Source: CAD feature listing. Evaluate the final solid. Frame: model axes, mm. A direction names the side the tool comes from. Coordinates: 2 decimals unless noted, no trailing zeros. Write each loop counter-clockwise with the first axis right and the second up, starting at its lowest first coordinate (ties: lowest second). Pieces come first, ordered by that corner, then holes. Notation, with made-up numbers: M 6,74 L 65,74 A19 cw 65,110 Z; hole C -15,11 d2. An arc over 180 degrees is marked long. One line per item, written item: value. Start each with the question number.
Item 1: Mould query, pull axis Z, two halves, no side actions, for faces 3 (the cylindrical face through (12.88, 20.11, 6.33)), 4 (the flat face through (0, 0, 0)), 5 (the cylindrical face through (3.131, 9.175, -0.43)). Classes: released by +Z, released by -Z, zero draft, split by the parting line, or undercut.
Item 2: Cut plane A-A, the plane z = 0. Output: boundary loops of the cut face in (x, y), then the cut area to 3 significant figures.
Item 3: Cut plane D-D, the plane x = 2. Output: boundary loops of the cut face in (y, z).
Item 4: Ray query, L1, parallel to Y at x = 7, z = -19; L2, parallel to Z at x = 11.5, y = 18 (3 decimals). Return the intervals inside material, ascending. Write a range as from..to.
Item 5: Pin query (flat end, axial travel): P1, Ø6, axis at x = 10, z = -3.5, coming from the +Y side; P2, Ø4, axis at x = 9, y = -11.5, coming from the +Z side; P3, Ø3, axis at y = -11.11, z = 0, coming from the -X side. Return the tip coordinate at first contact, or that it passes through.
Item 6: Cut plane C-C, the plane x = 23. Output: boundary loops of the cut face in (y, z), then the cut area to 3 significant figures.
Item 7: Set-up query: faces 1 (the cylindrical face through (3.13, 0.09, 9.13)), 2 (the flat face through (25.4, 0, 0)). Return all of +Z, -Z, +X, -X, +Y, -Y with unobstructed straight access to the full face (end or side cutting, diameter ignored); none if empty.
```python
from build123d import *

# Parameters (mm, degrees)
SKETCH1_W          = 25.4
SKETCH1_H          = 21.082
SKETCH2_R          = 1.984375
CUT_EXTRUDE1_DEPTH = 6.35


with BuildPart() as part:
    # Sketch1 → Revolve1 (revolve)
    with BuildSketch(Plane.XY):
        with Locations((12.7, 10.541)):
            Rectangle(SKETCH1_W, SKETCH1_H)
    revolve(axis=Axis((-29.670962963, 0, 0), (1, 0, 0)))

    # Sketch2 → Cut-Extrude1 (cut)
    with BuildSketch(Plane.ZY):
        with Locations((0, 11.1125)):
            Circle(SKETCH2_R)
        with Locations((11.1125, 0)):
            Circle(SKETCH2_R)
        with Locations((0, -11.1125)):
            Circle(SKETCH2_R)
        with Locations((-11.1125, 0)):
            Circle(SKETCH2_R)
    extrude(amount=-CUT_EXTRUDE1_DEPTH, mode=Mode.SUBTRACT)


solid = part.part
```
From the geometry:
1. face 3: split by the parting line
1. face 4: zero draft
1. face 5: undercut
2. outline: M 0,-21.08 L 25.4,-21.08 L 25.4,21.08 L 0,21.08 L 0,13.1 L 6.35,13.1 L 6.35,9.13 L 0,9.13 L 0,-9.13 L 6.35,-9.13 L 6.35,-13.1 L 0,-13.1 Z
2. area: 1,020 mm²
3. outline: C 0,0 d42.16; hole C -11.11,0 d3.97; hole C 0,-11.11 d3.97; hole C 0,11.11 d3.97; hole C 11.11,0 d3.97
4. L1: y = -9.14..9.14
4. L2: z = -10.975..10.975
5. P1: stops at y = 21.08
5. P2: stops at z = 18.82
5. P3: stops at x = 6.35
6. outline: C 0,0 d42.16
6. area: 1,400 mm²
7. face 1: -X
7. face 2: +Z, -Z, +X, +Y, -Y
